Build history of the part. All positions in model axes, mm. A direction names the side the tool comes from. Coordinates: 2 decimals unless noted, no trailing zeros. Write each loop counter-clockwise with the first axis right and the second up, starting at its lowest first coordinate (ties: lowest second). Pieces come first, ordered by that corner, then holes. Notation, with made-up numbers: (-1.75, 28.25) -> (21.25, 28.25) arc R29 cw to (21.25, 49.25) -> close; hole circle Ø2 at (68, 61). An arc over 180 degrees is marked (long way). Write each question's results on one line, items separated by ' | '. Start each with the question number.
Q1. Saw through at A-A on x = -68.25. Give the cut face in (y, z), and give its area (3 significant figures).
Q2. Drop flat-ended pins along their axis: pin 1 Ø3 at (x, y) = (-68.59, -90) entering from +Z; pin 2 Ø1.5 at (y, z) = (-87.5, -8.5) entering from -X; pin 3 Ø2 at (x, z) = (-67, -0.5) entering from -Y. Give the stop position or say it passes through.
Q3. Saw through at C-C on z = -4. Give the cut face in (x, y), and give its area (3 significant figures).
Q4. Drill centre lines: line 1 (Z direction, x = -66.5, y = -86.75); line 2 (X direction, y = -89.5, z = 2.5); line 3 (X direction, y = -88.75, z = 0.25). Where is each one in solid material? Low to high.
Q5. Saw through at B-B on y = -90. Give the cut face in (x, z), and give its area (3 significant figures).
Q6. Tool access for faces 1 (the face through (-70, -92, -5)), 2 (the face through (-68.91, -87.52, 0.45)): list every direction of +Z, -Z, +X, -X, +Y, -Y with a clear straight run to the whole face (end or side of a thin tool).
Q7. Saw through at D-D on z = 3. Give the cut face in (x, y), and give its area (3 significant figures).
Q8. Two-plate mould, pull along X, no slides. Class faces 3 (the face through (-69, -90, -10)), 4 (the face through (-70.43, -93.55, -3.99)), 5 (the face through (-69, -90, -1)): released by +X, released by -X, zero draft, split by the parting line, or undercut.
from build123d import *

# Parameters (mm, degrees)
BOSS_EXTRUDE1_DEPTH      = 4
BOSS_EXTRUDE1_DEPTH_BACK = 3
SKETCH1_R                = 2.5
SKETCH2_R                = 4
BOSS_EXTRUDE2_DEPTH      = 2
SKETCH3_R                = 2
CUT_EXTRUDE1_DEPTH       = 5
SKETCH4_R                = 2
BOSS_EXTRUDE3_DEPTH      = 5


with BuildPart() as part:
    # Sketch1 → Boss-Extrude1 (new, two sides: drawn at the far end of the back side and taken through both)
    with BuildSketch(Plane.XY.offset(-BOSS_EXTRUDE1_DEPTH_BACK)):
        with Locations((-68.585871194, -90)):
            Circle(SKETCH1_R)
    extrude(amount=BOSS_EXTRUDE1_DEPTH + BOSS_EXTRUDE1_DEPTH_BACK)

    # Sketch2 → Boss-Extrude2 (add)
    with BuildSketch(Plane(origin=(0, 0, -3), x_dir=(-1, 0, 0), z_dir=(0, 0, -1))):
        with Locations((68.585871194, -90)):
            Circle(SKETCH2_R)
    extrude(amount=BOSS_EXTRUDE2_DEPTH)

    # Sketch3 → Cut-Extrude1 (cut)
    with BuildSketch(Plane.XY.offset(4)):
        with Locations((-68.585871194, -90)):
            Circle(SKETCH3_R)
    extrude(amount=-CUT_EXTRUDE1_DEPTH, mode=Mode.SUBTRACT)

    # Sketch4 → Boss-Extrude3 (add)
    with BuildSketch(Plane(origin=(0, 0, -5), x_dir=(-1, 0, 0), z_dir=(0, 0, -1))):
        with Locations(Location((68.585871194, -90, 0), (0, 0, 180))):
            Circle(SKETCH4_R)
    extrude(amount=BOSS_EXTRUDE3_DEPTH)


solid = part.part
Returned:
1) outline: (-93.99, -5) -> (-91.97, -5) -> (-91.97, -10) -> (-88.03, -10) -> (-88.03, -5) -> (-86.01, -5) -> (-86.01, -3) -> (-87.52, -3) -> (-87.52, 4) -> (-88.03, 4) -> (-88.03, -1) -> (-91.97, -1) -> (-91.97, 4) -> (-92.48, 4) -> (-92.48, -3) -> (-93.99, -3) -> close | area: 50.6 mm2
2) pin 1: stops at z = -1 | pin 2: stops at x = -69.55 | pin 3: stops at y = -92.43
3) outline: circle Ø8 at (-68.59, -90) | area: 50.3 mm2
4) line 1: z = -5 to -3 | line 2: x = -71.04 to -70.52, -66.65 to -66.14 | line 3: x = -70.75 to -70.15, -67.02 to -66.42
5) outline: (-72.59, -5) -> (-70.59, -5) -> (-70.59, -10) -> (-66.59, -10) -> (-66.59, -5) -> (-64.59, -5) -> (-64.59, -3) -> (-66.09, -3) -> (-66.09, 4) -> (-66.59, 4) -> (-66.59, -1) -> (-70.59, -1) -> (-70.59, 4) -> (-71.09, 4) -> (-71.09, -3) -> (-72.59, -3) -> close | area: 51.0 mm2
6) face 1: -Z | face 2: +Z
7) outline: circle Ø5 at (-68.59, -90); hole circle Ø4 at (-68.59, -90) | area: 7.07 mm2
8) face 3: zero draft | face 4: split by the parting line | face 5: undercut
